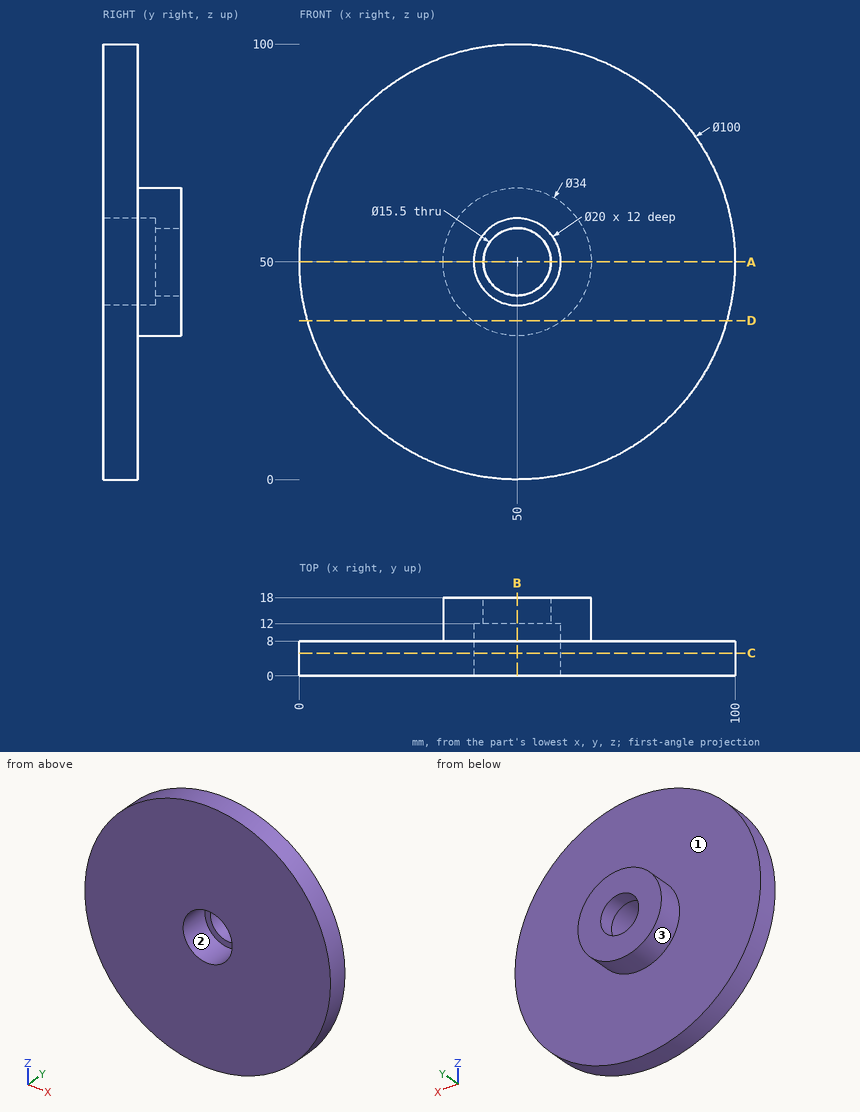
Answer from the drawing. Dimensions are ordinates in mm from the lowest x, y and z of the part. Give positions to 0.01 mm unless a question says otherwise; leave off trailing zeros. Order: outer loops, then holes, each group sorted by start corner. A loop starts at its lowest first (then second) coordinate and runs counter-clockwise, first axis right, second up. Notation, with made-up numbers: (-38, -39.75) - (-26, -39.75) arc R19 cw to (-26, -11.75) - close; hole circle Ø11 at (80.25, 39.25). An arc over 180 degrees is marked (long way). One line per item, written item: value. Start each with the question number.
1. Section A-A, the plane z = 50 is taken. Write down the section's boundary in (x, y), then the cut area to 3 significant figures.
2. For a pull along X with two mould halves and no side action, classify the marked faces 1, 2 and 3 as released by +X, released by -X, zero draft, split by the parting line, or undercut.
3. Section D-D, the plane z = 36.5 is taken. Write down the section's boundary in (x, y).
4. Section B-B, the plane x = 50 is taken. Write down the section's boundary in (y, z).
5. Consider line 1 (Z direction, x = 50, y = 6.5); line 2 (Y direction, x = 81.5, z = 32); line 3 (X direction, y = 13, z = 43). Determine where each line is inside the solid, lowest interval first.
6. Section C-C, the plane y = 5.25 is taken. Write down the section's boundary in (x, z), then the cut area to 3 significant figures.
7. Each of these flat-tipped pins is pushed along its axis until it touches: pin 1 Ø3 at (y, z) = (8.5, 81) entering from +X; pin 2 Ø1 at (x, y) = (20, 7) entering from -Z; pin 3 Ø5 at (x, z) = (78, 70.5) entering from +Y; pin 4 Ø12 at (x, z) = (50, 50) entering from -Y. Where does it stop, or does it pass through?
Filled sheet:
1. outline: (0, 0) - (40, 0) - (40, 12) - (42.25, 12) - (42.25, 18) - (33, 18) - (33, 8) - (0, 8) - close; (57.75, 12) - (60, 12) - (60, 0) - (100, 0) - (100, 8) - (67, 8) - (67, 18) - (57.75, 18) - close
1. area: 807 mm²
2. face 1: zero draft
2. face 2: undercut
2. face 3: split by the parting line
3. outline: (1.86, 0) - (98.14, 0) - (98.14, 8) - (60.33, 8) - (60.33, 18) - (39.67, 18) - (39.67, 8) - (1.86, 8) - close
4. outline: (0, 0) - (8, 0) - (8, 33) - (18, 33) - (18, 42.25) - (12, 42.25) - (12, 40) - (0, 40) - close; (0, 60) - (12, 60) - (12, 57.75) - (18, 57.75) - (18, 67) - (8, 67) - (8, 100) - (0, 100) - close
5. line 1: 0 to 40, 60 to 100
5. line 2: 0 to 8
5. line 3: 34.51 to 46.67, 53.33 to 65.49
6. outline: circle Ø100 at (50, 50); hole circle Ø20 at (50, 50)
6. area: 7,540 mm²
7. pin 1: x = 90.31
7. pin 2: z = 9.63
7. pin 3: y = 8
7. pin 4: through
